Can you work these out from the drawing? Everything is in mm from the part's minimum corner. A direction names the side the tool comes from. Round coordinates to 2 decimals unless told otherwise and drop trailing zeros. Order: outer loops, then holes, each group sorted by start corner. A loop starts at its lowest first (then second) coordinate and runs counter-clockwise, first axis right, second up. Notation, with made-up numbers: (-6, 49) - (5, 49) arc R34 cw to (5, 82) - close; hole circle Ø7 at (-2, 64). An arc over 180 degrees is marked (long way). Write item = value, one per line.
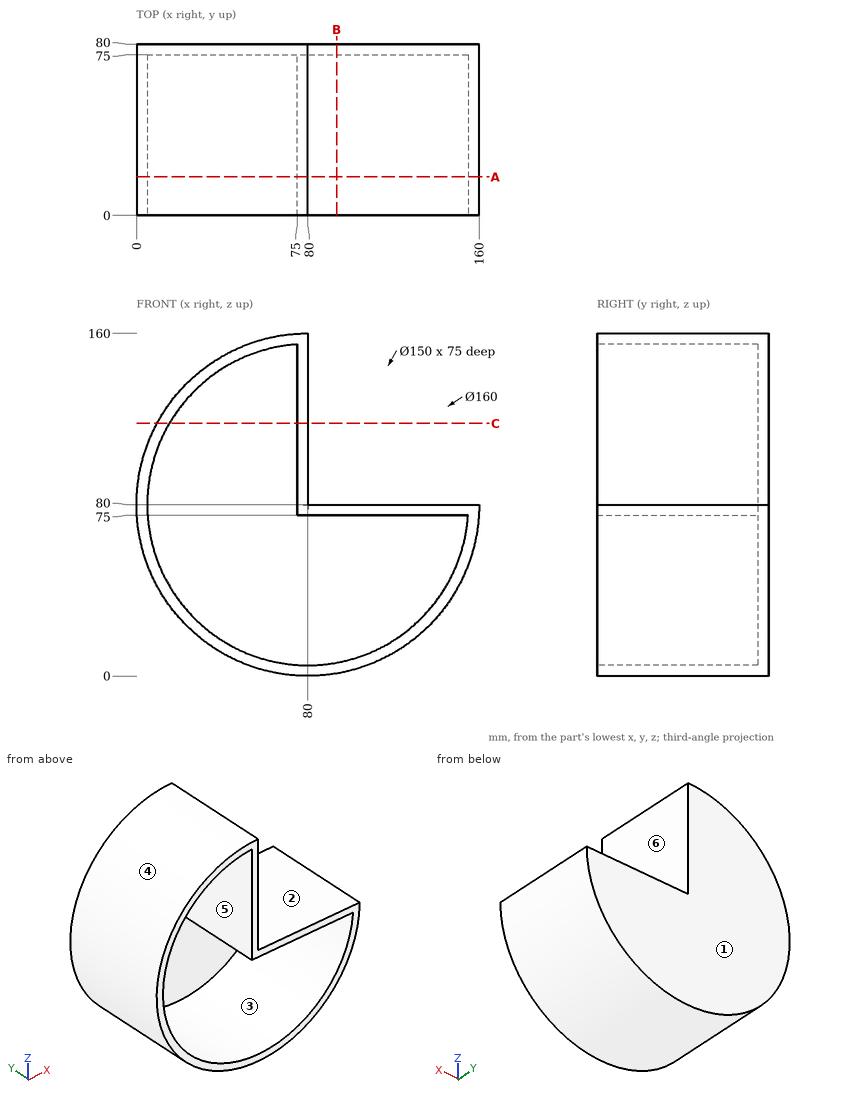
(1) Thinking about a two-plate mould opening in X: for the marked faces 4, 5 and 6, which applies, +X half, -X half, draft (parallel to the pull), parting line (faces both ways), or undercut?
Computed:
face_4 = parting line
face_5 = undercut
face_6 = +X half
(2) If we section it at B-B (x = 93.5): Write out the boundary of the cut face in (y, z) (3 decimals), plus the area to 3 significant figures.
Computed:
outline = (0, 1.147) - (80, 1.147) - (80, 80) - (0, 80) - (0, 75) - (75, 75) - (75, 6.225) - (0, 6.225) - close
area = 1,150 mm^2
(3) If we section it at A-A (y = 18): Write out the boundary of the cut face in (x, z).
Computed:
outline = (80, 80) - (80, 160) arc R80 ccw (long way) to (160, 80) - close; hole (75, 75) - (75, 154.83) arc R75 ccw (long way) to (154.83, 75) - close
(4) If I drill on line 1 (X direction, y = 13, z = 82.5); line 2 (Y direction, x = 47.5, z = 124); line 3 (X direction, y = 64, z = 32.5), over which ranges is the centre line in solid material (lowest first)? Write a range as from..to.
Computed:
line_1 = 0.04..5.04, 75..80
line_2 = 75..80
line_3 = 15.63..21.96, 138.04..144.37
(5) If we section it at C-C (z = 118): Write out the boundary of the cut face in (x, y).
Computed:
outline = (9.6, 0) - (15.34, 0) - (15.34, 75) - (75, 75) - (75, 0) - (80, 0) - (80, 80) - (9.6, 80) - close
(6) Will these pins go through, and if not, where does the flat tip stop? P1, Ø4, axis at x = 127.5, y = 28, coming from the -Z side; P2, Ø24, axis at x = 124, y = 58, coming from the +Z side; P3, Ø8, axis at x = 27.5, y = 61.5, coming from the -Z side.
Computed:
P1 = 14.2
P2 = 80
P3 = 16.38
(7) On a 3-axis mill with a long thin cutter (end or side, diameter ignored), from which of +Z, -Z, +X, -X, +Y, -Y can I reach the whole of each face in a straight line? I mean the marked faces 1, 2 and 3. Say none if no direction works.
Computed:
face_1 = +Z, -Z, +X, -X, +Y
face_2 = +Z, +X, +Y, -Y
face_3 = -Y
